Part model, mm, in its own coordinate system. A direction names the side the tool comes from. Give positions to 0.01 mm unless a question says otherwise; leave off trailing zeros. Loops run counter-clockwise (first coordinate to the right, second up) from the corner with the lowest first, then second, coordinate; pieces in that order, holes last. Notation, with made-up numbers: (41.25, 12.25) -> (90.25, 12.25) arc R32 ccw to (90.25, 44.25) -> close; hole circle Ø9 at (-0.75, 50). An arc over 180 degrees is marked (long way). Write item = value, one per line.
from build123d import *

# Parameters (mm, degrees)
BOSS_EXTRUDE1_DEPTH = 5
FILLET1_R           = 1


with BuildPart() as part:
    # Sketch1 → Boss-Extrude1 (new body)
    with BuildSketch(Plane.XY):
        Polygon((42.02, -4.628401452), (37.437424305, -6.628401452), (45.397424305, -24.867052718), (49.98, -22.867052718), (52, -27.49545417), (52, -32.49545417), (47, -32.49545417), (0, -5), (0, 0), (4.95, 0), (4.95, 5), (35.05, 5), (35.05, 0), (40, 0), align=None)
    extrude(amount=BOSS_EXTRUDE1_DEPTH)

    # Fillet1
    fillet1_edges = [part.edges().sort_by_distance(p)[0] for p in [
        (4.95, 5, 2.5),
        (35.05, 5, 2.5),
        (40, 0, 2.5),
        (42.02, -4.628401452, 2.5),
        (49.98, -22.867052718, 2.5),
        (52, -27.49545417, 2.5),
        (52, -32.49545417, 2.5),
        (47, -32.49545417, 2.5),
        (0, -5, 2.5),
    ]]
    fillet(fillet1_edges, radius=FILLET1_R)


solid = part.part
1) Pull direction Y, two halves, no side cores. Call faces 5 (the face through (41.63, -4.49, 2.54)), 6 (the face through (41.36, -15.62, 2.46)), 7 (the face through (4.95, 2, 2)), 8 (the face through (47.2, -24.08, 2.46)): pulls with the +Y half, pulls with the -Y half, needs draft (parallel to the pull), parting line crosses it, or undercut.
Resolved:
face_5 = undercut
face_6 = undercut
face_7 = needs draft
face_8 = pulls with the +Y half
2) Slice it at B-B, the plane x = 24.5. List the corners of the cut face in (y, z), and give its area (3 significant figures).
Resolved:
outline = (-19.33, 0) -> (5, 0) -> (5, 5) -> (-19.33, 5) -> close
area = 122 mm²
3) Drop flat-ended pins along their axis: P1, Ø1.5, axis at y = -24, z = 4.5, coming from the -X side; P2, Ø2.5, axis at x = 2.5, z = 2.5, coming from the +Y side; P3, Ø3, axis at y = 2, z = 3, coming from the +X side; P4, Ø6, axis at x = 9, y = -16.5, coming from the -Z side. Give the stop position or say it passes through.
Resolved:
P1 = 31.2
P2 = 0
P3 = 35.05
P4 = through
4) Slice it at C-C, the plane y = -28.5. List the corners of the cut face in (x, z), and give its area (3 significant figures).
Resolved:
outline = (40.17, 0) -> (52, 0) -> (52, 5) -> (40.17, 5) -> close
area = 59.1 mm²
5) Drill centre lines: line 1 along Y through (x, z) = (42.5, 4.3); line 2 along Y through (x, z) = (41.5, 2.6); line 3 along Y through (x, z) = (17, 1.6). Where is each one in solid material? Low to high. Write a range as [from, to].
Resolved:
line_1 = [-29.86, -18.23]
line_2 = [-29.28, -15.94], [-4.72, -3.44]
line_3 = [-14.95, 5]
6) Slice it at A-A, the plane z = 0.65. List the corners of the cut face in (x, y).
Resolved:
outline = (0, -4.43) arc R1 ccw to (0.5, -5.29) -> (46.77, -32.36) arc R1 ccw to (47.27, -32.5) -> (51, -32.5) arc R1 ccw to (52, -31.5) -> (52, -27.7) arc R1 ccw to (51.92, -27.3) -> (50.38, -23.78) arc R1 ccw to (49.06, -23.27) -> (45.4, -24.87) -> (37.44, -6.63) -> (41.1, -5.03) arc R1 ccw to (41.62, -3.71) -> (40.26, -0.6) arc R1 ccw to (39.35, 0) -> (35.05, 0) -> (35.05, 4) arc R1 ccw to (34.05, 5) -> (5.95, 5) arc R1 ccw to (4.95, 4) -> (4.95, 0) -> (0, 0) -> close
7) Which spindle directions (+Z, -Z, +X, -X, +Y, -Y) get a long thin tool onto all of the face, cutting with end or side? Do faces 1 (the face through (2, 0, 2)), 2 (the face through (39.296, -5.817, 2.465)), 3 (the face through (20, 5, 2)), 4 (the face through (37, 0, 2)). Say none if no direction does.
Resolved:
face_1 = +Z, -Z, -X, +Y
face_2 = +Z, -Z, +X
face_3 = +Z, -Z, +X, -X, +Y
face_4 = +Z, -Z, +X, +Y
